Geometry check sheet. Reference: drawing and pictorial views, mm from the part's lowest x, y, z. A direction names the side the tool comes from. Round coordinates to 2 decimals unless told otherwise and drop trailing zeros. Write each loop counter-clockwise with the first axis right and the second up, starting at its lowest first coordinate (ties: lowest second). Pieces come first, ordered by that corner, then holes. Notation, with made-up numbers: M 33,51 L 65,51 A5 ccw 65,58 Z; hole C -1.5,24.5 d6. An arc over 180 degrees is marked long. One line per item, written item: value. Start each with the question number.
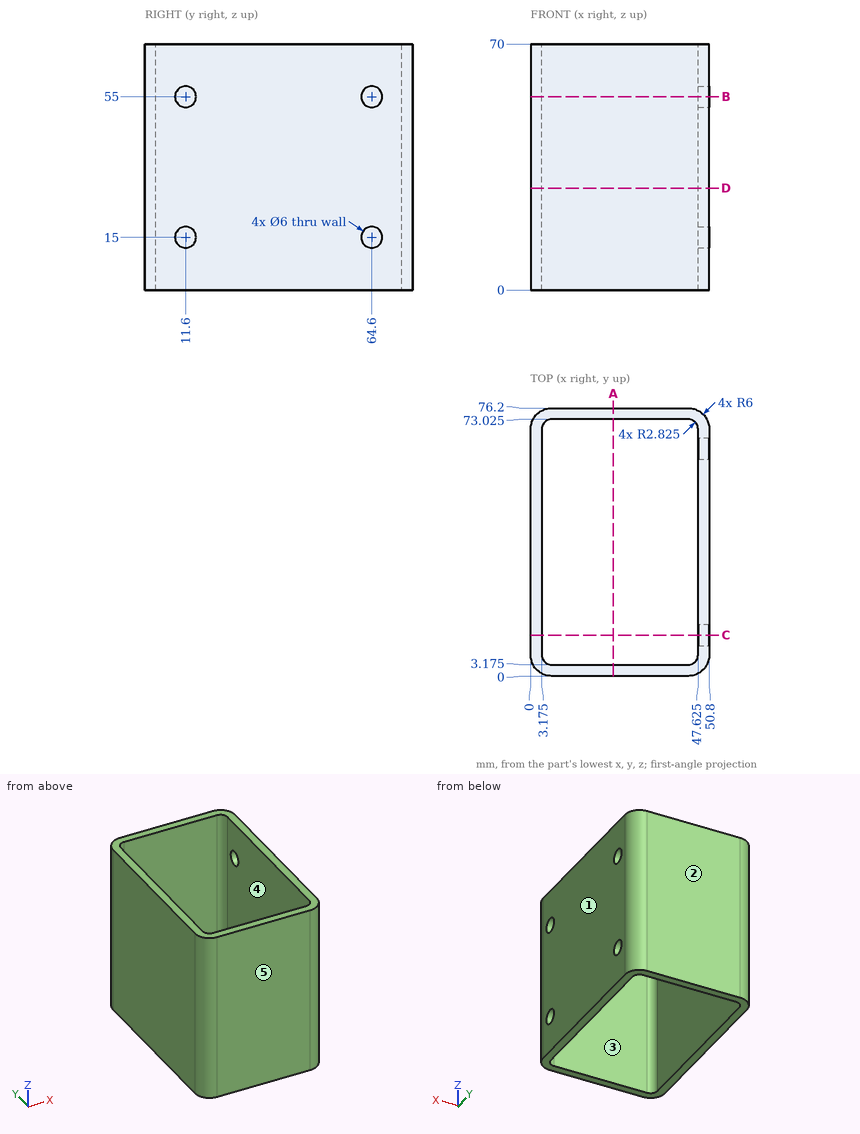
1) Gauge pin test, flat ends, axial feed: pin 1 Ø10 at (x, y) = (40.5, 59) entering from +Z; pin 2 Ø5 at (y, z) = (11.6, 55) entering from +X (3 decimals). Record the tip position at first contact, or that the pin passes through.
2) Cross-section at C-C (y = 11.6). Record the boundary of the cut face in (x, z) (3 decimals), then the cut area to 3 significant figures.
3) Access from +Z, -Z, +X, -X, +Y, -Y to the whole of each face (thin tool, end or side, straight path). Record for the marked faces 4 and 5.
4) Cross-section at D-D (z = 29). Record the boundary of the cut face in (x, y) (3 decimals).
5) Mould release check, pull along Y, two halves, no side actions. Record for the marked faces 1, 2 and 3: pulls with the +Y half, pulls with the -Y half, needs draft (parallel to the pull), parting line crosses it, or undercut.
6) Thickness scan on line 1 (X direction, y = 60, z = 40.5) (3 decimals); line 2 (Z direction, x = 48.6, y = 11.6); line 3 (Y direction, x = 43, z = 36) (3 decimals). Record the ranges inside material, lowest first.
7) Cross-section at A-A (x = 23.5). Record the boundary of the cut face in (y, z) (3 decimals), then the cut area to 4 significant figures.
8) Cross-section at B-B (z = 55). Record the boundary of the cut face in (x, y) (3 decimals), then the cut area to 3 significant figures.
Results below:
1. pin 1: passes through
1. pin 2: stops at x = 3.175
2. outline: M 0,0 L 3.175,0 L 3.175,70 L 0,70 Z; M 47.625,0 L 50.8,0 L 50.8,12 L 47.625,12 Z; M 47.625,18 L 50.8,18 L 50.8,52 L 47.625,52 Z; M 47.625,58 L 50.8,58 L 50.8,70 L 47.625,70 Z
2. area: 406 mm²
3. face 4: +Z, -Z
3. face 5: +Z, -Z, +X, -X, -Y
4. outline: M 0,6 A6 ccw 6,0 L 44.8,0 A6 ccw 50.8,6 L 50.8,70.2 A6 ccw 44.8,76.2 L 6,76.2 A6 ccw 0,70.2 Z; hole M 3.175,6 A2.825 ccw 6,3.175 L 44.8,3.175 A2.825 ccw 47.625,6 L 47.625,70.2 A2.825 ccw 44.8,73.025 L 6,73.025 A2.825 ccw 3.175,70.2 Z
5. face 1: needs draft
5. face 2: pulls with the +Y half
5. face 3: undercut
6. line 1: x = 0 to 3.175, 47.625 to 50.8
6. line 2: z = 0 to 12, 18 to 52, 58 to 70
6. line 3: y = 0 to 3.175, 73.025 to 76.2
7. outline: M 0,0 L 3.175,0 L 3.175,70 L 0,70 Z; M 73.025,0 L 76.2,0 L 76.2,70 L 73.025,70 Z
7. area: 444.5 mm²
8. outline: M 0,6 A6 ccw 6,0 L 44.8,0 A6 ccw 50.8,6 L 50.8,8.6 L 47.625,8.6 L 47.625,6 A2.825 cw 44.8,3.175 L 6,3.175 A2.825 cw 3.175,6 L 3.175,70.2 A2.825 cw 6,73.025 L 44.8,73.025 A2.825 cw 47.625,70.2 L 47.625,67.6 L 50.8,67.6 L 50.8,70.2 A6 ccw 44.8,76.2 L 6,76.2 A6 ccw 0,70.2 Z; M 47.625,14.6 L 50.8,14.6 L 50.8,61.6 L 47.625,61.6 Z
8. area: 704 mm²
